Build history of the part. All positions in model axes, mm. Give positions to 0.01 mm unless a question says otherwise; leave off trailing zeros. Loops run counter-clockwise (first coordinate to the right, second up) from the corner with the lowest first, then second, coordinate; pieces in that order, holes last. Notation, with made-up numbers: (34.25, 28) -> (64.25, 28) arc R17 ccw to (64.25, 57) -> close; hole circle Ø8 at (-16.75, 69). An arc over 180 degrees is marked (long way). One line per question, with ' | ' between items. Start each with the question number.
(1) Flat gauge pins, fed straight in: pin 1 Ø16.5 at (x, y) = (117.8, -57.75) entering from -Z; pin 2 Ø5 at (x, y) = (117.8, -57.75) entering from +Z; pin 3 Ø5.5 at (x, y) = (-15.5, -61.5) entering from -Z. Where does each tip first touch, or does it go through?
(2) Slice it at A-A, the plane y = 37.5. Write the cut outline in (x, z), then the cut area to 3 significant figures.
(3) Slice it at B-B, the plane z = 1.75. Give the number of separate pieces and of enclosed holes in the cut face, then the cut area to 3 significant figures.
(4) Drill centre lines: L1, parallel to X at y = -57.75, z = 7.55; L2, parallel to X at y = -57.75, z = 2.7; L3, parallel to Y at x = 14, z = 7.75. Where is each one in solid material? Low to high. Write a range as from..to.
```python
from build123d import *

# Parameters (mm, degrees)
SKETCH1_W                      = 240.6
SKETCH1_H                      = 180.2
BOSS_EXTRUDE1_DEPTH            = 8
SKETCH2_W                      = 160.6
SKETCH2_H                      = 100.2
CUT_EXTRUDE1_DEPTH             = 200.503872501
CUT_EXTRUDE2_DEPTH             = 7
CUT_EXTRUDE3_DEPTH             = 7
CUT_EXTRUDE4_DEPTH             = 7
CUT_EXTRUDE5_DEPTH             = 7
F_6_5_6_5_DIAMETER_HOLE1_D     = 6.5
F_6_5_6_5_DIAMETER_HOLE1_DEPTH = 8
SKETCH9_R                      = 9.267416037
SKETCH9_R_2                    = 9.269178346
SKETCH9_R_3                    = 9.266671768
CUT_EXTRUDE7_DEPTH             = 4


with BuildPart() as part:
    # Sketch1 → Boss-Extrude1 (new body)
    with BuildSketch(Plane(origin=(0, 0, 0), x_dir=(-1, 0, 0), z_dir=(0, 0, -1))):
        with Locations((-50.702318109, 12.34999924)):
            Rectangle(SKETCH1_W, SKETCH1_H)
    extrude(amount=-BOSS_EXTRUDE1_DEPTH)

    # Sketch2 → Cut-Extrude1 (cut, through all)
    with BuildSketch(Plane.XY.offset(8)):
        with Locations((50.702318109, 12.34999924)):
            Rectangle(SKETCH2_W, SKETCH2_H)
    extrude(amount=-CUT_EXTRUDE1_DEPTH, mode=Mode.SUBTRACT)

    # Sketch3 → Cut-Extrude2 (cut)
    with BuildSketch(Plane(origin=(0, 0, 0), x_dir=(-1, 0, 0), z_dir=(0, 0, -1))):
        Polygon((-117.686768689, -48.483328992), (-127.060792146, -58.198146757), (-117.921667286, -67.016672528), (-108.547643828, -57.301854763), align=None)
    extrude(amount=-CUT_EXTRUDE2_DEPTH, mode=Mode.SUBTRACT)

    # Sketch4 → Cut-Extrude3 (cut)
    with BuildSketch(Plane(origin=(0, 0, 0), x_dir=(-1, 0, 0), z_dir=(0, 0, -1))):
        Polygon((6.939207854, -58.198146757), (16.078332714, -67.016672528), (25.452356172, -57.301854763), (16.313231311, -48.483328992), align=None)
    extrude(amount=-CUT_EXTRUDE3_DEPTH, mode=Mode.SUBTRACT)

    # Sketch5 → Cut-Extrude4 (cut)
    with BuildSketch(Plane(origin=(0, 0, 0), x_dir=(-1, 0, 0), z_dir=(0, 0, -1))):
        Polygon((-37.727458813, -58.198146757), (-28.588333952, -67.016672528), (-19.214310494, -57.301854763), (-28.353435355, -48.483328992), align=None)
    extrude(amount=-CUT_EXTRUDE4_DEPTH, mode=Mode.SUBTRACT)

    # Sketch6 → Cut-Extrude5 (cut)
    with BuildSketch(Plane(origin=(0, 0, 0), x_dir=(-1, 0, 0), z_dir=(0, 0, -1))):
        Polygon((-82.39412548, -58.198146757), (-73.255000619, -67.016672528), (-63.880977161, -57.301854763), (-73.020102022, -48.483328992), align=None)
    extrude(amount=-CUT_EXTRUDE5_DEPTH, mode=Mode.SUBTRACT)

    # Ø6.5 (6.5) Diameter Hole1
    with Locations(Plane.XY.offset(8)):
        with Locations((117.804217987, -57.75000076), (-16.097681891, -57.75000076), (28.568984776, -57.75000076), (73.235651442, -57.75000076)):
            Hole(F_6_5_6_5_DIAMETER_HOLE1_D / 2, depth=F_6_5_6_5_DIAMETER_HOLE1_DEPTH)

    # Sketch9 → Cut-Extrude7 (cut)
    with BuildSketch(Plane(origin=(0, 0, 0), x_dir=(-1, 0, 0), z_dir=(0, 0, -1))):
        with Locations((-117.804217987, -57.75000076)):
            Circle(SKETCH9_R)
        with Locations((-73.235651442, -57.75000076)):
            Circle(SKETCH9_R_2)
        with Locations((-28.568984776, -57.75000076)):
            Circle(SKETCH9_R_2)
        with Locations((16.097681891, -57.75000076)):
            Circle(SKETCH9_R_3)
    extrude(amount=-CUT_EXTRUDE7_DEPTH, mode=Mode.SUBTRACT)


solid = part.part
```
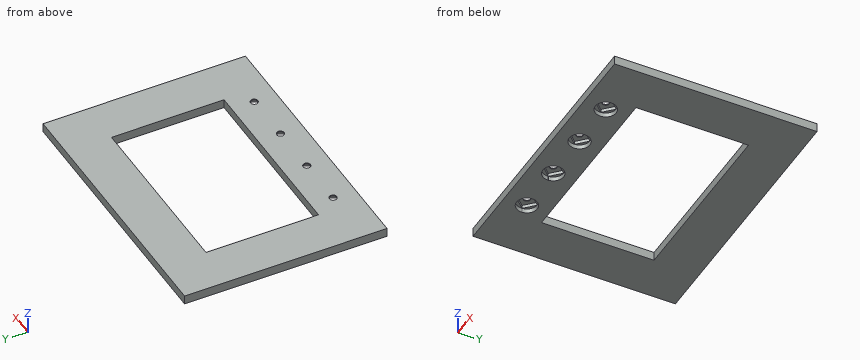
Final values:
1) pin 1: z = 4 | pin 2: through | pin 3: z = 7
2) outline: (-69.6, 0) -> (-29.6, 0) -> (-29.6, 8) -> (-69.6, 8) -> close; (131, 0) -> (171, 0) -> (171, 8) -> (131, 8) -> close | area: 640 mm2
3) separate pieces: 1 | enclosed holes: 5 | area: 26,200 mm2
4) L1: -69.6..-19.35, -12.85..25.32, 31.82..69.99, 76.49..114.55, 121.05..171 | L2: -69.6..-25.36, -6.83..19.3, 37.84..63.97, 82.5..108.54, 127.07..171 | L3: -77.75..-37.75, 62.45..102.45
